The listing builds one solid part. Answer for the finished solid, in the listing's coordinates (mm). A direction names the side the tool comes from. Round coordinates to 2 decimals unless told otherwise and drop trailing zeros. Write each loop counter-clockwise with the first axis right and the second up, starting at its lowest first coordinate (ties: lowest second). Pieces come first, ordered by that corner, then holes.
Item 1: Find section B-B on z = 5.5. Give the vertices of the cut face in (x, y).
Item 2: For a pull along Y with two mould halves and no side action, classify faces 1 (the face through (-15.4, -9.43, 17.52)), 2 (the face through (-16.797, -13.859, 10.14)), 3 (the face through (-12, 15, 10)) as +Y half, -Y half, draft (parallel to the pull), parting line (faces both ways), or undercut.
Item 3: Find section D-D on x = 5.5. Give the vertices of the cut face in (y, z).
Item 4: Find section C-C on y = 5.5. Give the vertices of the cut face in (x, z), then the cut area to 3 significant figures.
Item 5: A tool of negligible diameter and unlimited length cuts with its end or side. For faces 4 (the face through (12, 15, 10)), 5 (the face through (0, 5, 10)), 6 (the face through (8, -5, 18)), from which of +Z, -Z, +X, -X, +Y, -Y can it reach the whole face along a straight path? Write none if from no direction.
Item 6: Find section A-A on x = 12.5. Give the vertices of the cut face in (y, z).
Item 7: Find the intervals of material crossed by probe 1 along X at (y, z) = (10, 2); probe 2 along Y at (x, z) = (-1.5, 14.5); probe 3 along Z at (x, y) = (7, -8.75), in increasing order.
Item 8: Each of these flat-tipped pins is pushed along its axis until it touches: pin 1 (5 mm diameter, centred on x = -2.5, y = -4, fed in from -Z); pin 2 (3 mm diameter, centred on x = 6, z = 14.5, fed in from +Y). Where does it stop, or does it pass through?
```python
from build123d import *

# Parameters (mm, degrees)
BOSS_EXTRUDE1_DEPTH = 20
SKETCH5_W           = 10.2
SKETCH5_H           = 10.2
CUT_EXTRUDE2_DEPTH  = 44.829214002
SKETCH6_W           = 8
SKETCH6_H           = 10
CUT_EXTRUDE3_DEPTH  = 31.805843601
FILLET1_R           = 2
FILLET3_R           = 4
FILLET4_R           = 4


with BuildPart() as part:
    # Sketch1 → Boss-Extrude1 (new body)
    with BuildSketch(Plane.XY):
        Polygon((-10, 15), (-10, 5), (10, 5), (10, 15), (18, 15), (18, -15), (-18, -15), (-18, 15), align=None)
    extrude(amount=BOSS_EXTRUDE1_DEPTH)

    # Sketch5 → Cut-Extrude2 (cut, through all)
    with BuildSketch(Plane.ZY.offset(18)):
        with Locations((10, -4.9)):
            Rectangle(SKETCH5_W, SKETCH5_H)
    extrude(amount=-CUT_EXTRUDE2_DEPTH, mode=Mode.SUBTRACT)

    # Sketch6 → Cut-Extrude3 (cut, through all)
    with BuildSketch(Plane.XY.offset(20)):
        with Locations((0, -5)):
            Rectangle(SKETCH6_W, SKETCH6_H)
        with Locations((-12, -5)):
            Rectangle(SKETCH6_W, SKETCH6_H)
        with Locations((12, -5)):
            Rectangle(SKETCH6_W, SKETCH6_H)
    extrude(amount=-CUT_EXTRUDE3_DEPTH, mode=Mode.SUBTRACT)

    # Fillet1
    fillet1_edges = [part.edges().sort_by_distance(p)[0] for p in [
        (16, 0, 17.55),
        (16, 0, 2.45),
        (16, -10, 17.55),
        (16, -10, 2.45),
        (8, -10, 17.55),
        (8, -10, 2.45),
        (8, 0, 17.55),
        (8, 0, 2.45),
        (-4, -10, 17.55),
        (-4, -10, 2.45),
        (-4, 0, 17.55),
        (-4, 0, 2.45),
        (4, 0, 17.55),
        (4, 0, 2.45),
        (4, -10, 17.55),
        (4, -10, 2.45),
        (-16, -10, 17.55),
        (-16, -10, 2.45),
        (-16, 0, 17.55),
        (-16, 0, 2.45),
        (-8, 0, 17.55),
        (-8, 0, 2.45),
        (-8, -10, 17.55),
        (-8, -10, 2.45),
    ]]
    fillet(fillet1_edges, radius=FILLET1_R)

    # Fillet3
    fillet3_edges = [part.edges().sort_by_distance(p)[0] for p in [
        (0, -15, 0),
        (18, -15, 10),
        (-18, -15, 10),
        (0, -15, 20),
    ]]
    fillet(fillet3_edges, radius=FILLET3_R)

    # Fillet4
    fillet4_edges = [part.edges().sort_by_distance(p)[0] for p in [
        (18, 15, 10),
        (-18, 15, 10),
    ]]
    fillet(fillet4_edges, radius=FILLET4_R)


solid = part.part
```
Check values:
1. outline: (-18, -11) arc R4 ccw to (-14, -15) - (14, -15) arc R4 ccw to (18, -11) - (18, -10) - (-18, -10) - close; (-18, 0.2) - (18, 0.2) - (18, 11) arc R4 ccw to (14, 15) - (10, 15) - (10, 5) - (-10, 5) - (-10, 15) - (-14, 15) arc R4 ccw to (-18, 11) - close
2. face 1: undercut
2. face 2: -Y half
2. face 3: +Y half
3. outline: (-15, 4) arc R4 ccw to (-11, 0) - (5, 0) - (5, 20) - (-11, 20) arc R4 ccw to (-15, 16) - close; hole (-10, 4.9) - (0.2, 4.9) - (0.2, 15.1) - (-10, 15.1) - close
4. outline: (-18, 0) - (-10, 0) - (-10, 20) - (-18, 20) - close; (10, 0) - (18, 0) - (18, 20) - (10, 20) - close
4. area: 320 mm2
5. face 4: +Z, -Z, +X, -X, +Y
5. face 5: +Z, -Z, +Y
5. face 6: +Z, -Z
6. outline: (-15, 4) arc R4 ccw to (-11, 0) - (-10, 0) - (-10, 20) - (-11, 20) arc R4 ccw to (-15, 16) - close; (0, 0) - (15, 0) - (15, 20) - (0, 20) - (0, 15.1) - (0.2, 15.1) - (0.2, 4.9) - (0, 4.9) - close
7. probe 1: x = -18 to -10, 10 to 18
7. probe 2: y = -15 to -10, 0.2 to 5
7. probe 3: z = 0 to 4.9, 15.1 to 20
8. pin 1: stops at z = 0
8. pin 2: stops at y = 5
